Model file for the job. Use its own axes, mm. Face numbers are marked on the shaded views. A direction names the side the tool comes from. Give positions to 0.01 mm unless a question says otherwise; leave off trailing zeros. Loops run counter-clockwise (first coordinate to the right, second up) from the corner with the lowest first, then second, coordinate; pieces in that order, holes last. Notation, with made-up numbers: M 38,60.5 L 92,60.5 A22 cw 92,75.5 Z; hole C 68,-11 d2. An arc over 180 degrees is marked long. Answer in a Markdown table with one row per item.
```python
from build123d import *

# Parameters (mm, degrees)
BOSS_EXTRUDE2_DEPTH = 39.5


with BuildPart() as part:
    # Sketch6 → Boss-Extrude2 (new body, symmetric)
    with BuildSketch(Plane(origin=(0, 0, 0), x_dir=(0, 0, -1), z_dir=(1, 0, 0))):
        Polygon((-85.742753648, -14.325502792), (-88.841702167, -5.325502792), (-88.841702167, 10.674497208), (-57.649472482, 47.674497208), (76.526626639, 47.674497208), (88.425634479, 18.292332188), (91.510658272, 10.674497208), (91.510658272, -14.325502792), (94.010658272, -14.325502792), (94.010658272, -29.325502792), (-80.44551992, -29.325502792), (-91.235932802, -29.325502792), (-93.189341728, -23.652391339), (-93.189341728, -14.325502792), align=None)
    extrude(amount=BOSS_EXTRUDE2_DEPTH, both=True)


solid = part.part
```
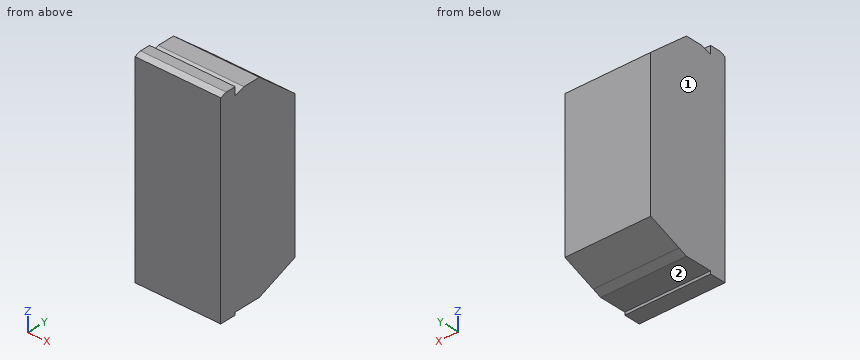
(1) Saw through at C-C, the plane y = 30.5. Give the cut face in (x, z), and give its area (3 significant figures).
Established:
| item | result |
|---|---|
| outline | M -39.5,-83.48 L 39.5,-83.48 L 39.5,72.13 L -39.5,72.13 Z |
| area | 12,300 mm2 |
(2) Saw through at A-A, the plane x = -8.5. Give the cut face in (y, z).
Established:
| item | result |
|---|---|
| outline | M -29.33,-94.01 L -14.33,-94.01 L -14.33,-91.51 L 10.67,-91.51 L 47.67,-76.53 L 47.67,57.65 L 10.67,88.84 L -5.33,88.84 L -14.33,85.74 L -14.33,93.19 L -23.65,93.19 L -29.33,91.24 Z |
(3) Wall check: L1, parallel to Z at x = 30, y = 3.5; L2, parallel to Z at x = -6, y = -13.5; L3, parallel to Y at x = 13.5, z = 60. Give the ranges that are in metal, low to high.
Established:
| item | result |
|---|---|
| L1 | z = -91.51 to 88.84 |
| L2 | z = -91.51 to 86.03 |
| L3 | y = -29.33 to 44.89 |
(4) Saw through at B-B, the plane y = -1.5. Give the cut face in (x, z).
Established:
| item | result |
|---|---|
| outline | M -39.5,-91.51 L 39.5,-91.51 L 39.5,88.84 L -39.5,88.84 Z |
(5) Flat gauge pins, fed straight in: P1, Ø5, axis at x = 15, y = 7, coming from the -Z side; P2, Ø6, axis at x = 16, y = 23.5, coming from the -Z side; P3, Ø2, axis at x = -18, z = 89, coming from the +Y side. Where does each tip first touch, or does it go through?
Established:
| item | result |
|---|---|
| P1 | stops at z = -91.51 |
| P2 | stops at z = -87.53 |
| P3 | stops at y = 11.67 |
(6) Which spindle directions (+Z, -Z, +X, -X, +Y, -Y) get a long thin tool onto all of the face, cutting with end or side? Do the marked faces 1 and 2. Say none if no direction does.
Established:
| item | result |
|---|---|
| face 1 | +Z, -Z, -X, +Y, -Y |
| face 2 | -Z, +X, -X, +Y |
